Geometry: final body of the model. Coordinates: model frame, mm. Face numbers are marked on the shaded views. A direction names the side the tool comes from. Give positions to 0.01 mm unless a question says otherwise; leave off trailing zeros. Write each loop counter-clockwise with the first axis right and the second up, starting at its lowest first coordinate (ties: lowest second). Pieces come first, ordered by that corner, then holes. Notation, with made-up numbers: M -12.5,3 L 17.5,3 A8 ccw 17.5,10 Z; hole C 43,39.25 d11. An arc over 180 degrees is marked long. Answer as a JSON object with one key per item and string values.
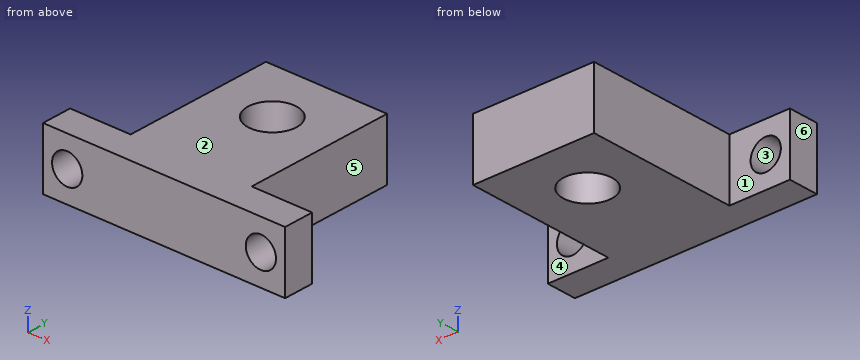
from build123d import *

# Parameters (mm, degrees)
RESSALTO_EXTRUS_O1_DEPTH      = 5
RESSALTO_EXTRUS_O1_DEPTH_BACK = 5
CORTE_EXTRUS_O1_DEPTH         = 5
CORTE_EXTRUS_O1_DEPTH_BACK    = 5
ESBO_O2_R                     = 4
ESBO_O3_R                     = 2.5
CORTE_EXTRUS_O2_DEPTH         = 29.722813233


with BuildPart() as part:
    # Esbo_o1 → Ressalto-extrus_o1 (new, two sides: drawn at the far end of the back side and taken through both)
    with BuildSketch(Plane.XY.offset(-RESSALTO_EXTRUS_O1_DEPTH_BACK)):
        Polygon((-10, 10), (-10, -15), (-20, -15), (-20, -20), (20, -20), (20, -15), (10, -15), (10, 10), align=None)
    extrude(amount=RESSALTO_EXTRUS_O1_DEPTH + RESSALTO_EXTRUS_O1_DEPTH_BACK)

    # Esbo_o2 → Corte-extrus_o1 (cut, two sides: drawn at the far end of the back side and taken through both)
    with BuildSketch(Plane.XY.offset(-CORTE_EXTRUS_O1_DEPTH_BACK)):
        Circle(ESBO_O2_R)
    extrude(amount=CORTE_EXTRUS_O1_DEPTH + CORTE_EXTRUS_O1_DEPTH_BACK, mode=Mode.SUBTRACT)

    # Esbo_o3 → Corte-extrus_o2 (cut, through all)
    with BuildSketch(Plane(origin=(0, 0, 0), x_dir=(1, 0, 0), z_dir=(0, 1, 0))):
        with Locations(Location((-16, 0, 0), (0, 0, 270))):
            Circle(ESBO_O3_R)
        with Locations(Location((16, 0, 0), (0, 0, 270))):
            Circle(ESBO_O3_R)
    extrude(amount=-CORTE_EXTRUS_O2_DEPTH, mode=Mode.SUBTRACT)


solid = part.part
1) Cut plane B-B on x = 0. Return loops of the section in (y, z).
Geometry check:
{"outline": "M -20,-5 L -4,-5 L -4,5 L -20,5 Z; M 4,-5 L 10,-5 L 10,5 L 4,5 Z"}
2) Cut plane D-D on z = -4. Return loops of the section in (x, y), and give its area (3 significant figures).
Geometry check:
{"outline": "M -20,-20 L 20,-20 L 20,-15 L 10,-15 L 10,10 L -10,10 L -10,-15 L -20,-15 Z; hole C 0,0 d8", "area": "650 mm2"}
3) Line query: line 1 (X direction, y = -16.6, z = 0); line 2 (Y direction, x = 0, z = 0); line 3 (X direction, y = -13.5, z = -3.5). Output: solid intervals per line, ascending. Write a range as from..to.
Geometry check:
{"line 1": "x = -20..-18.5, -13.5..13.5, 18.5..20", "line 2": "y = -20..-4, 4..10", "line 3": "x = -10..10"}
4) Contact query for flat-ended pins moving along their axis: P1, Ø13, axis at x = 0, y = 0, coming from the +Z side; P2, Ø1.5, axis at y = -9, z = 1, coming from the +X side; P3, Ø5, axis at y = -2, z = 0, coming from the -X side; P4, Ø3, axis at x = 14, z = -2, coming from the +Y side. Output: stop coordinate, or through.
Geometry check:
{"P1": "stops at z = 5", "P2": "stops at x = 10", "P3": "stops at x = -10", "P4": "stops at y = -15"}
5) Cut plane A-A on z = 0. Return loops of the section in (x, y), and give its area (3 significant figures).
Geometry check:
{"outline": "M -20,-20 L -18.5,-20 L -18.5,-15 L -20,-15 Z; M -13.5,-20 L 13.5,-20 L 13.5,-15 L 10,-15 L 10,10 L -10,10 L -10,-15 L -13.5,-15 Z; M 18.5,-20 L 20,-20 L 20,-15 L 18.5,-15 Z; hole C 0,0 d8", "area": "600 mm2"}
6) Pull-direction query (X, two-part tool) for the marked faces 3, 4, 5 and 6; classes: pulls with the +X half, pulls with the -X half, needs draft (parallel to the pull), parting line crosses it, or undercut.
Geometry check:
{"face 3": "undercut", "face 4": "needs draft", "face 5": "pulls with the +X half", "face 6": "pulls with the -X half"}
7) Cut plane C-C on y = 0. Return loops of the section in (x, z), and give its area (3 significant figures).
Geometry check:
{"outline": "M -10,-5 L -4,-5 L -4,5 L -10,5 Z; M 4,-5 L 10,-5 L 10,5 L 4,5 Z", "area": "120 mm2"}
8) Set-up query: the marked faces 1 and 2. Return all of +Z, -Z, +X, -X, +Y, -Y with unobstructed straight access to the full face (end or side cutting, diameter ignored); none if empty.
Geometry check:
{"face 1": "+Z, -Z, -X, +Y", "face 2": "+Z, +X, -X, +Y, -Y"}
